from build123d import *

# Parameters (mm, degrees)
EXTRUDE_THIN1_DEPTH                               = 425
SKETCH2_R                                         = 1
SKETCH2_R_2                                       = 15.187
CUT_EXTRUDE1_DEPTH                                = 10
SKETCH3_R                                         = 2.195
CUT_EXTRUDE2_DEPTH                                = 458.71088036
CSK_FOR_4_FLAT_HEAD_MACHINE_SCREW_100_D           = 3.2639
CSK_FOR_4_FLAT_HEAD_MACHINE_SCREW_100_DEPTH       = 10
CSK_FOR_4_FLAT_HEAD_MACHINE_SCREW_100_CSINK_D     = 5.715
CSK_FOR_4_FLAT_HEAD_MACHINE_SCREW_100_CSINK_ANGLE = 100
CSK_FOR_4_FLAT_HEAD_MACHINE_SCREW_100_TIP         = 0.980574487
CSK_FOR_M3_FLAT_HEAD_MACHINE_SCREW1_D             = 3.4
CSK_FOR_M3_FLAT_HEAD_MACHINE_SCREW1_DEPTH         = 10
CSK_FOR_M3_FLAT_HEAD_MACHINE_SCREW1_CSINK_D       = 6.3
CSK_FOR_M3_FLAT_HEAD_MACHINE_SCREW1_CSINK_ANGLE   = 90
CSK_FOR_M3_FLAT_HEAD_MACHINE_SCREW1_TIP           = 1.021463052


with BuildPart() as part:
    # Sketch1 → Extrude-Thin1 (new body)
    with BuildSketch(Plane(origin=(0, 0, 0), x_dir=(1, 0, 0), z_dir=(0, 1, 0))):
        with BuildLine():
            Line((-84.75, 12), (-84.75, 1.5))
            ThreePointArc((-84.75, 1.5), (-84.310660172, 0.439339828), (-83.25, 0))
            Line((-83.25, 0), (83.25, 0))
            ThreePointArc((83.25, 0), (84.310660172, 0.439339828), (84.75, 1.5))
            Line((84.75, 1.5), (84.75, 12))
            Line((84.75, 12), (82.75, 12))
            Line((82.75, 12), (82.75, 2))
            Line((82.75, 2), (-82.75, 2))
            Line((-82.75, 2), (-82.75, 12))
            Line((-82.75, 12), (-84.75, 12))
        make_face()
    extrude(amount=EXTRUDE_THIN1_DEPTH)

    # Sketch2 → Cut-Extrude1 (cut)
    with BuildSketch(Plane(origin=(0, 0, -2), x_dir=(-1, 0, 0), z_dir=(0, 0, -1))):
        with Locations((-60.5, 376.25)):
            Circle(SKETCH2_R)
        with Locations((11, 376.25)):
            Circle(SKETCH2_R)
        with Locations((-60.5, 304.75)):
            Circle(SKETCH2_R)
        with Locations((11, 304.75)):
            Circle(SKETCH2_R)
        with Locations((45, 22)):
            Circle(SKETCH2_R_2)
        with Locations((-45, 22)):
            Circle(SKETCH2_R_2)
        with Locations((-59.2875, 7.7125)):
            Circle(SKETCH2_R)
        with Locations((-30.7125, 7.7125)):
            Circle(SKETCH2_R)
        with Locations((-30.7125, 36.2875)):
            Circle(SKETCH2_R)
        with Locations((-59.2875, 36.2875)):
            Circle(SKETCH2_R)
        with Locations((30.7125, 36.2875)):
            Circle(SKETCH2_R)
        with Locations((59.2875, 36.2875)):
            Circle(SKETCH2_R)
        with Locations((59.2875, 7.7125)):
            Circle(SKETCH2_R)
        with Locations((30.7125, 7.7125)):
            Circle(SKETCH2_R)
        with BuildLine():
            Line((-60.75, 342.5), (-41.75, 342.5))
            ThreePointArc((-41.75, 342.5), (-39.75, 340.5), (-41.75, 338.5))
            Line((-41.75, 338.5), (-60.75, 338.5))
            ThreePointArc((-60.75, 338.5), (-62.75, 340.5), (-60.75, 342.5))
        make_face()
        with BuildLine():
            Line((-7.75, 342.5), (11.25, 342.5))
            ThreePointArc((11.25, 342.5), (13.25, 340.5), (11.25, 338.5))
            Line((11.25, 338.5), (-7.75, 338.5))
            ThreePointArc((-7.75, 338.5), (-9.75, 340.5), (-7.75, 342.5))
        make_face()
        with BuildLine():
            Line((-60.062887166, 349.5), (-40.241933385, 349.5))
            ThreePointArc((-40.241933385, 349.5), (-38.241933385, 347.5), (-40.241933385, 345.5))
            Line((-40.241933385, 345.5), (-60.062887166, 345.5))
            ThreePointArc((-60.062887166, 345.5), (-62.062887166, 347.5), (-60.062887166, 349.5))
        make_face()
        with BuildLine():
            Line((-57.916247904, 356.5), (-34.393650761, 356.5))
            ThreePointArc((-34.393650761, 356.5), (-32.393650761, 354.5), (-34.393650761, 352.5))
            Line((-34.393650761, 352.5), (-57.916247904, 352.5))
            ThreePointArc((-57.916247904, 352.5), (-59.916247904, 354.5), (-57.916247904, 356.5))
        make_face()
        with BuildLine():
            Line((-9.258066615, 349.5), (10.562887166, 349.5))
            ThreePointArc((10.562887166, 349.5), (12.562887166, 347.5), (10.562887166, 345.5))
            Line((10.562887166, 345.5), (-9.258066615, 345.5))
            ThreePointArc((-9.258066615, 345.5), (-11.258066615, 347.5), (-9.258066615, 349.5))
        make_face()
        with BuildLine():
            Line((-15.106349239, 356.5), (8.416247904, 356.5))
            ThreePointArc((8.416247904, 356.5), (10.416247904, 354.5), (8.416247904, 352.5))
            Line((8.416247904, 352.5), (-15.106349239, 352.5))
            ThreePointArc((-15.106349239, 352.5), (-17.106349239, 354.5), (-15.106349239, 356.5))
        make_face()
        with BuildLine():
            Line((-9.258066615, 335.5), (10.562887166, 335.5))
            ThreePointArc((10.562887166, 335.5), (12.562887166, 333.5), (10.562887166, 331.5))
            Line((10.562887166, 331.5), (-9.258066615, 331.5))
            ThreePointArc((-9.258066615, 331.5), (-11.258066615, 333.5), (-9.258066615, 335.5))
        make_face()
        with BuildLine():
            Line((-15.106349239, 328.5), (8.416247904, 328.5))
            ThreePointArc((8.416247904, 328.5), (10.416247904, 326.5), (8.416247904, 324.5))
            Line((8.416247904, 324.5), (-15.106349239, 324.5))
            ThreePointArc((-15.106349239, 324.5), (-17.106349239, 326.5), (-15.106349239, 328.5))
        make_face()
        with BuildLine():
            Line((-60.062887166, 335.5), (-40.241933385, 335.5))
            ThreePointArc((-40.241933385, 335.5), (-38.241933385, 333.5), (-40.241933385, 331.5))
            Line((-40.241933385, 331.5), (-60.062887166, 331.5))
            ThreePointArc((-60.062887166, 331.5), (-62.062887166, 333.5), (-60.062887166, 335.5))
        make_face()
        with BuildLine():
            Line((-57.916247904, 328.5), (-34.393650761, 328.5))
            ThreePointArc((-34.393650761, 328.5), (-32.393650761, 326.5), (-34.393650761, 324.5))
            Line((-34.393650761, 324.5), (-57.916247904, 324.5))
            ThreePointArc((-57.916247904, 324.5), (-59.916247904, 326.5), (-57.916247904, 328.5))
        make_face()
        with BuildLine():
            Line((-53.990383034, 363.5), (4.490383034, 363.5))
            ThreePointArc((4.490383034, 363.5), (6.490383034, 361.5), (4.490383034, 359.5))
            Line((4.490383034, 359.5), (-53.990383034, 359.5))
            ThreePointArc((-53.990383034, 359.5), (-55.990383034, 361.5), (-53.990383034, 363.5))
        make_face()
        with BuildLine():
            Line((-47.377416998, 370.5), (-2.122583002, 370.5))
            ThreePointArc((-2.122583002, 370.5), (-0.122583002, 368.5), (-2.122583002, 366.5))
            Line((-2.122583002, 366.5), (-47.377416998, 366.5))
            ThreePointArc((-47.377416998, 366.5), (-49.377416998, 368.5), (-47.377416998, 370.5))
        make_face()
        with BuildLine():
            Line((-37.25, 377.5), (-12.25, 377.5))
            ThreePointArc((-12.25, 377.5), (-10.25, 375.5), (-12.25, 373.5))
            Line((-12.25, 373.5), (-37.25, 373.5))
            ThreePointArc((-37.25, 373.5), (-39.25, 375.5), (-37.25, 377.5))
        make_face()
        with BuildLine():
            Line((-53.990383034, 321.5), (4.490383034, 321.5))
            ThreePointArc((4.490383034, 321.5), (6.490383034, 319.5), (4.490383034, 317.5))
            Line((4.490383034, 317.5), (-53.990383034, 317.5))
            ThreePointArc((-53.990383034, 317.5), (-55.990383034, 319.5), (-53.990383034, 321.5))
        make_face()
        with BuildLine():
            Line((-47.377416998, 314.5), (-2.122583002, 314.5))
            ThreePointArc((-2.122583002, 314.5), (-0.122583002, 312.5), (-2.122583002, 310.5))
            Line((-2.122583002, 310.5), (-47.377416998, 310.5))
            ThreePointArc((-47.377416998, 310.5), (-49.377416998, 312.5), (-47.377416998, 314.5))
        make_face()
        with BuildLine():
            Line((-37.25, 307.5), (-12.25, 307.5))
            ThreePointArc((-12.25, 307.5), (-10.25, 305.5), (-12.25, 303.5))
            Line((-12.25, 303.5), (-37.25, 303.5))
            ThreePointArc((-37.25, 303.5), (-39.25, 305.5), (-37.25, 307.5))
        make_face()
    extrude(amount=-CUT_EXTRUDE1_DEPTH, mode=Mode.SUBTRACT)

    # Sketch3 → Cut-Extrude2 (cut, through all)
    with BuildSketch(Plane.ZY.offset(84.75)):
        with Locations((-7, 367.5)):
            Circle(SKETCH3_R)
        with Locations((-7, 212.5)):
            Circle(SKETCH3_R)
        with Locations((-7, 47.5)):
            Circle(SKETCH3_R)
    extrude(amount=-CUT_EXTRUDE2_DEPTH, mode=Mode.SUBTRACT)

    # CSK for #4 Flat Head Machine Screw (100)1
    with Locations(Plane.XY):
        with Locations((-59.2875, 36.2875), (-59.2875, 7.7125), (-30.7125, 7.7125), (-30.7125, 36.2875), (30.7125, 36.2875), (59.2875, 36.2875), (59.2875, 7.7125), (30.7125, 7.7125)):
            CounterSinkHole(CSK_FOR_4_FLAT_HEAD_MACHINE_SCREW_100_D / 2, CSK_FOR_4_FLAT_HEAD_MACHINE_SCREW_100_CSINK_D / 2, depth=CSK_FOR_4_FLAT_HEAD_MACHINE_SCREW_100_DEPTH, counter_sink_angle=CSK_FOR_4_FLAT_HEAD_MACHINE_SCREW_100_CSINK_ANGLE)
            with Locations((0, 0, -(CSK_FOR_4_FLAT_HEAD_MACHINE_SCREW_100_DEPTH + CSK_FOR_4_FLAT_HEAD_MACHINE_SCREW_100_TIP / 2))):  # 118° drill point
                Cone(0, CSK_FOR_4_FLAT_HEAD_MACHINE_SCREW_100_D / 2, CSK_FOR_4_FLAT_HEAD_MACHINE_SCREW_100_TIP, mode=Mode.SUBTRACT)

    # CSK for M3 Flat Head Machine Screw1
    with Locations(Plane.XY):
        with Locations((-11, 376.25), (60.5, 376.25), (60.5, 304.75), (-11, 304.75)):
            CounterSinkHole(CSK_FOR_M3_FLAT_HEAD_MACHINE_SCREW1_D / 2, CSK_FOR_M3_FLAT_HEAD_MACHINE_SCREW1_CSINK_D / 2, depth=CSK_FOR_M3_FLAT_HEAD_MACHINE_SCREW1_DEPTH, counter_sink_angle=CSK_FOR_M3_FLAT_HEAD_MACHINE_SCREW1_CSINK_ANGLE)
            with Locations((0, 0, -(CSK_FOR_M3_FLAT_HEAD_MACHINE_SCREW1_DEPTH + CSK_FOR_M3_FLAT_HEAD_MACHINE_SCREW1_TIP / 2))):  # 118° drill point
                Cone(0, CSK_FOR_M3_FLAT_HEAD_MACHINE_SCREW1_D / 2, CSK_FOR_M3_FLAT_HEAD_MACHINE_SCREW1_TIP, mode=Mode.SUBTRACT)


solid = part.part
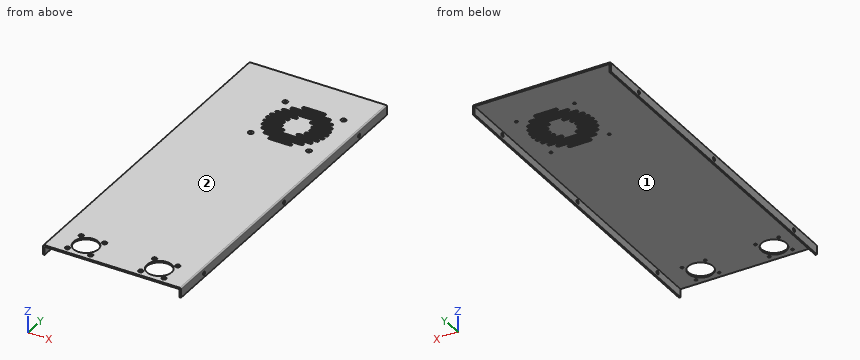
Source: CAD feature listing. Evaluate the final solid. Frame: model axes, mm. Face numbers are marked on the shaded views. Round coordinates to 2 decimals unless told otherwise and drop trailing zeros. Loops run counter-clockwise (first coordinate to the right, second up) from the corner with the lowest first, then second, coordinate; pieces in that order, holes last. Notation, with made-up numbers: M 70.25,55.5 L 118.25,55.5 A29 cw 118.25,76.5 Z; hole C 47,3 d6. An arc over 180 degrees is marked long. Return JSON: item names as keys, results as strings. Group by question number.
1. Pin query (flat end, axial travel): pin 1 (0.6 mm diameter, centred on x = 0, z = -1, fed in from -Y); pin 2 (4 mm diameter, centred on x = 52, z = -4.5, fed in from +Y); pin 3 (4 mm diameter, centred on x = -6, y = 79.5, fed in from -Z). Return the tip coordinate at first contact, or that it passes through.
2. Section query B-B on x = -45. Output: boundary loops of the cut face in (y, z), and give its area (3 significant figures).
3. Section query A-A on y = 22. Output: boundary loops of the cut face in (x, z).
4. Section query C-C on y = 241.5. Output: boundary loops of the cut face in (x, z), and give its area (3 significant figures).
5. Material intervals for line 1 along Y through (x, z) = (84.2, -7) (3 decimals); line 2 along Y through (x, z) = (-11, -1.7); line 3 along X through (y, z) = (304.75, -1.7), sorted ascending. Write a range as from..to.
6. Mould query, pull axis X, two halves, no side actions, for the marked faces 1 and 2. Classes: released by +X, released by -X, zero draft, split by the parting line, or undercut.
Checks:
{
 "1": {"pin 1": "stops at y = 0", "pin 2": "passes through", "pin 3": "stops at z = -2"},
 "2": {"outline": "M 0,-2 L 6.81,-2 L 6.81,0 L 0,0 Z; M 37.19,-2 L 425,-2 L 425,0 L 37.19,0 Z", "area": "789 mm²"},
 "3": {"outline": "M -84.75,-12 L -82.75,-12 L -82.75,-2 L -60.19,-2 L -60.19,0 L -83.25,0 A1.5 ccw -84.75,-1.5 Z; M -29.81,-2 L 29.81,-2 L 29.81,0 L -29.81,0 Z; M 60.19,-2 L 82.75,-2 L 82.75,-12 L 84.75,-12 L 84.75,-1.5 A1.5 ccw 83.25,0 L 60.19,0 Z"},
 "4": {"outline": "M -84.75,-12 L -82.75,-12 L -82.75,-2 L 82.75,-2 L 82.75,-12 L 84.75,-12 L 84.75,-1.5 A1.5 ccw 83.25,0 L -83.25,0 A1.5 ccw -84.75,-1.5 Z", "area": "378 mm²"},
 "5": {"line 1": "y = 0..45.305, 49.695..210.305, 214.695..365.305, 369.695..425", "line 2": "y = 0..303.05, 306.45..331.55, 335.45..338.5, 342.5..345.55, 349.45..374.55, 377.95..425", "line 3": "x = -84.75..-12.7, -9.3..10.4, 39.1..58.8, 62.2..84.75"},
 "6": {"face 1": "undercut", "face 2": "zero draft"}
}
